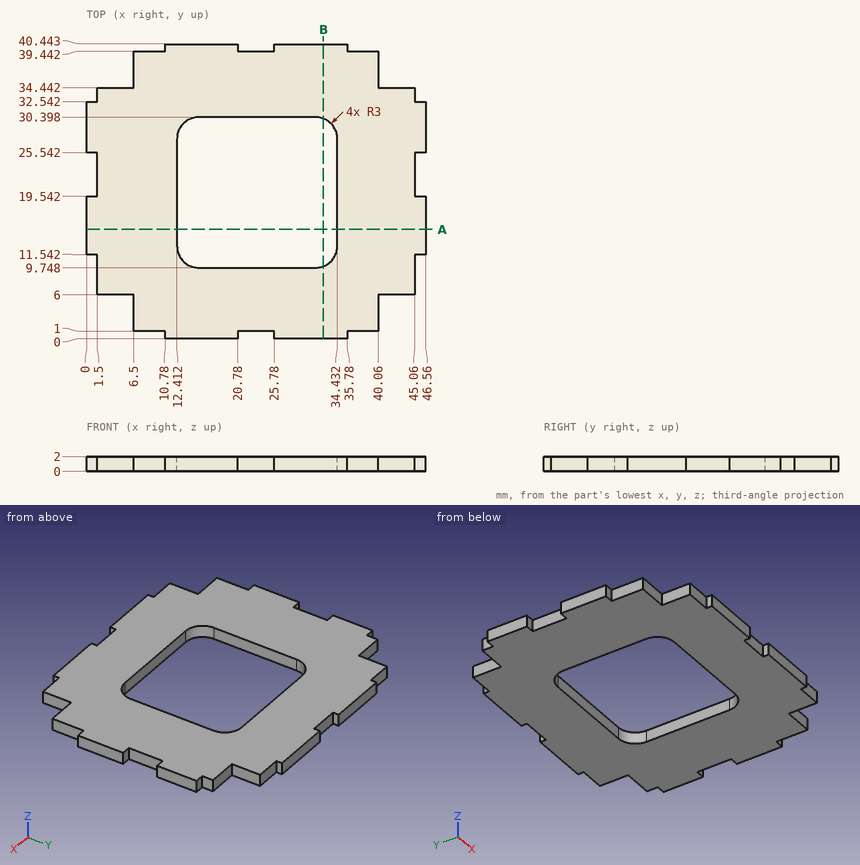
Print and shaded views of the part. All mm, measured from the part's lowest x, y and z. Round coordinates to 2 decimals unless told otherwise and drop trailing zeros. Write each loop counter-clockwise with the first axis right and the second up, starting at its lowest first coordinate (ties: lowest second). Pieces come first, ordered by that corner, then holes. Notation, with made-up numbers: M 38,-19 L 48,-19 A25 ccw 48,12 Z; hole C -30,85.25 d9. An arc over 180 degrees is marked long. One line per question, with ' | ' between items.
(1) Pin check, flat tips, straight feed: pin 1 (0.8 mm diameter, centred on x = 1, z = 1, fed in from -Y); pin 2 (1 mm diameter, centred on x = 38, z = 1, fed in from +Y); pin 3 (1 mm diameter, centred on y = 36.5, z = 0.5, fed in from -X). Stop position of each tip, or through.
Answer key:
pin 1: stops at y = 11.54 | pin 2: stops at y = 39.44 | pin 3: stops at x = 6.5
(2) Saw through at A-A on y = 15. Write the cut outline in (x, z).
Answer key:
outline: M 0,0 L 12.41,0 L 12.41,2 L 0,2 Z; M 34.43,0 L 46.56,0 L 46.56,2 L 34.43,2 Z
(3) Saw through at B-B on x = 32.5. Write the cut outline in (y, z) (1 decimal).
Answer key:
outline: M 0,0 L 9.9,0 L 9.9,2 L 0,2 Z; M 30.2,0 L 40.4,0 L 40.4,2 L 30.2,2 Z
(4) Probe line 1 along Y through (x, z) = (29, 0.7); line 2 along X through (y, z) = (24.5, 0.9); line 3 along X through (y, z) = (13, 0.2). List the from-to ranges inside material, lowest first.
Answer key:
line 1: y = 0 to 9.75, 30.4 to 40.44 | line 2: x = 1.5 to 12.41, 34.43 to 45.06 | line 3: x = 0 to 12.41, 34.43 to 46.56
